```python
from build123d import *

# Parameters (mm, degrees)
SKETCH1_R           = 33.8
SKETCH1_R_2         = 30
SKETCH1_R_3         = 25
SKETCH1_R_4         = 10
BOSS_EXTRUDE1_DEPTH = 6.5
SKETCH1_3_R         = 30
SKETCH1_3_R_2       = 25
BOSS_EXTRUDE2_DEPTH = 7.5
BOSS_EXTRUDE3_DEPTH = 6.5
CIRPATTERN1_COUNT   = 42


with BuildPart() as part:
    # Sketch1 → Boss-Extrude1 (new, symmetric)
    # profile 1 of 3: a face of its own
    with BuildSketch(Plane.YZ):
        with Locations(Location((0, 0, 0), (0, 0, 90))):
            Circle(SKETCH1_R)
        Circle(SKETCH1_R_2, mode=Mode.SUBTRACT)
    # profile 2 of 3: a face of its own
    with BuildSketch(Plane.YZ):
        Circle(SKETCH1_R_2)
        Circle(SKETCH1_R_3, mode=Mode.SUBTRACT)
    # profile 3 of 3: a face of its own
    with BuildSketch(Plane.YZ):
        Circle(SKETCH1_R_3)
        with Locations(Location((0, 0, 0), (0, 0, 90))):
            Circle(SKETCH1_R_4, mode=Mode.SUBTRACT)
    extrude(amount=BOSS_EXTRUDE1_DEPTH, both=True)

    # Sketch1_3 → Boss-Extrude2 (add, symmetric)
    with BuildSketch(Plane.YZ):
        with Locations(Location((0, 0, 0), (0, 0, 270))):
            Circle(SKETCH1_3_R)
        with Locations(Location((0, 0, 0), (0, 0, 270))):
            Circle(SKETCH1_3_R_2, mode=Mode.SUBTRACT)
    extrude(amount=BOSS_EXTRUDE2_DEPTH, both=True)

    # Sketch1_4 → Boss-Extrude3 (add, symmetric)
    with BuildSketch(Plane.YZ):
        with BuildLine():
            Line((-33.7621436, 1.599268434), (-37.8, 0.6))
            Line((-37.8, 0.6), (-37.8, -0.6))
            Line((-37.8, -0.6), (-33.7621436, -1.599268434))
            ThreePointArc((-33.7621436, -1.599268434), (-33.8, 0), (-33.7621436, 1.599268434))
        make_face()
    boss_extrude3 = extrude(amount=BOSS_EXTRUDE3_DEPTH, both=True)

    # CirPattern1: Boss-Extrude3 ×42 about axis
    cirpattern1_axis = Axis((0, 0, 0), (1, 0, 0))
    for i in range(1, CIRPATTERN1_COUNT):
        add(boss_extrude3.rotate(cirpattern1_axis, i * 360 / CIRPATTERN1_COUNT))


solid = part.part
```
The listing builds one solid part. Answer for the finished solid, in the listing's coordinates (mm). A direction names the side the tool comes from. Give positions to 0.01 mm unless a question says otherwise; leave off trailing zeros. Loops run counter-clockwise (first coordinate to the right, second up) from the corner with the lowest first, then second, coordinate; pieces in that order, holes last. Notation, with made-up numbers: M 24.5,11.25 L 59.5,11.25 A23 cw 59.5,46.25 Z; hole C 56.25,37.5 d7. An arc over 180 degrees is marked long. One line per item, written item: value.
Q1. A cutting plane is placed at A-A on y = 0. Determine the outline of the cut face in (x, z).
Working result:
outline: M -7.5,-30 L -6.5,-30 L -6.5,-33.8 L 6.5,-33.8 L 6.5,-30 L 7.5,-30 L 7.5,-25 L 6.5,-25 L 6.5,-10 L -6.5,-10 L -6.5,-25 L -7.5,-25 Z; M -7.5,25 L -6.5,25 L -6.5,10 L 6.5,10 L 6.5,25 L 7.5,25 L 7.5,30 L 6.5,30 L 6.5,33.8 L -6.5,33.8 L -6.5,30 L -7.5,30 Z
Q2. Flat-ended cylindrical pins translate along their axes: P1, Ø22.5, axis at y = 8.5, z = 7, coming from the +X side; P2, Ø2, axis at x = 3.5, z = 29, coming from the +Y side; P3, Ø1, axis at x = 3, y = 10.5, coming from the -Z side. Find the tip coordinate at first contact, or state that the pin passes through.
Working result:
P1: stops at x = 6.5
P2: stops at y = 24.04
P3: stops at z = -32.29
Q3. For faces 4 (the face through (0.091, 26.993, -23.556)), 5 (the face through (0.091, -26.961, -23.507)), 6 (the face through (0.091, -3.775, -35.57)), 7 (the face through (0.091, -18.835, -30.41)), 8 (the face through (0.091, 3.775, 35.57)), determine the directions among +Z, -Z, +X, -X, +Y, -Y from which every point of the face is accessible in a straight line to the end or side of a thin tool.
Working result:
face 4: +X, -X, +Y
face 5: +X, -X, -Y
face 6: -Z, +X, -X
face 7: +X, -X
face 8: +Z, +X, -X
Q4. Determine the mould class of faces 1 (the face through (-7.5, 25, 7)), 2 (the face through (0.091, -14.092, -32.877)), 3 (the face through (0.091, 30.164, 19.226)) for opening direction Y: +Y half, -Y half, draft (parallel to the pull), parting line (faces both ways), or undercut.
Working result:
face 1: draft
face 2: undercut
face 3: +Y half
Q5. Find the intervals of material crossed by line 1 (Y direction, x = 7.1, z = 0); line 2 (Y direction, x = 2, z = 0); line 3 (Y direction, x = -4.25, z = -28.5), in increasing order. Write a range as from..to.
Working result:
line 1: y = -30..-25, 25..30
line 2: y = -37.8..-10, 10..37.8
line 3: y = -23.73..-21.24, -18.28..18.28, 21.24..23.73
